Could you check a few things on this model? Use its own coordinates, in mm. A direction names the side the tool comes from. Coordinates: 2 decimals unless noted, no trailing zeros. Order: outer loops, then holes, each group sorted by start corner. A loop starts at its lowest first (then second) coordinate and runs counter-clockwise, first axis right, second up. Notation, with made-up numbers: (-29.75, -14.75) - (-5.75, -14.75) arc R16 cw to (-5.75, 9.25) - close; hole circle Ø1 at (87.25, 43). An arc over 180 degrees is marked (long way). One line per item, written item: value.
from build123d import *

# Parameters (mm, degrees)
SKETCH_1_R           = 1
EXTRUDE_1_DEPTH      = 4
EXTRUDE_START        = 4
SKETCH_2_R           = 1.732050808
EXTRUDE_2_DEPTH      = 5
EXTRUDE_3_DEPTH      = 0.75
EXTRUDE_3_DEPTH_BACK = 0.75
SKETCH_3_R           = 2.5


with BuildPart() as part:
    # 草图1 → 凸台-拉伸1 (new body)
    with BuildSketch(Plane.XY):
        Polygon((0.866025404, 1.5), (-0.866025404, 1.5), (-1.732050808, 0), (-0.866025404, -1.5), (0.866025404, -1.5), (1.732050808, 0), align=None)
        Circle(SKETCH_1_R, mode=Mode.SUBTRACT)
    extrude(amount=EXTRUDE_1_DEPTH)

    # 草图2 → 凸台-拉伸2 (add)
    with BuildSketch(Plane.XY.offset(EXTRUDE_START)):
        Circle(SKETCH_2_R)
    extrude(amount=EXTRUDE_2_DEPTH)

    # 草图3 → 凸台-拉伸3 (add, two sides: drawn at the far end of the back side and taken through both)
    with BuildSketch(Plane(origin=(0, 0, 0), x_dir=(1, 0, 0), z_dir=(0, 1, 0)).offset(-EXTRUDE_3_DEPTH_BACK)):
        with BuildLine():
            Line((-1.732050808, -9), (-3.661865884, -13.39042296))
            ThreePointArc((-3.661865884, -13.39042296), (0, -19), (3.661865884, -13.39042296))
            Line((3.661865884, -13.39042296), (1.732050808, -9))
            Line((1.732050808, -9), (-1.732050808, -9))
        make_face()
        with Locations(Location((0, -15, 0), (0, 0, 270))):
            Circle(SKETCH_3_R, mode=Mode.SUBTRACT)
    extrude(amount=EXTRUDE_3_DEPTH + EXTRUDE_3_DEPTH_BACK)

    # 草图4 → 切除-旋转2 (revolve, cut)
    with BuildSketch(Plane(origin=(0, 0, 0), x_dir=(0, 0, -1), z_dir=(1, 0, 0))):
        with BuildLine():
            Line((-15, -2.610076627), (-15, 2.610076627))
            ThreePointArc((-15, 2.610076627), (-17.610076627, 0), (-15, -2.610076627))
        make_face()
    revolve(axis=Axis((0, -2.610076627, 15), (0, 1, 0)), mode=Mode.SUBTRACT)


solid = part.part
Item 1: If I drill on probe 1 along Y at (x, z) = (0, 2); probe 2 along Z at (x, y) = (0.75, 0.25); probe 3 along X at (y, z) = (-0.6, 14), over which ranges is the centre line in solid material (lowest first)?
Conclusion:
probe 1: -1.5 to -1, 1 to 1.5
probe 2: 4 to 12.51, 17.49 to 18.93
probe 3: -3.87 to -2.34, 2.34 to 3.87
Item 2: I want a section at B-B on z = 15. Please give me the cut outline in (x, y).
Conclusion:
outline: (-4, -0.75) - (-2.5, -0.75) arc R2.61 cw to (-2.5, 0.75) - (-4, 0.75) - close; (2.5, -0.75) - (4, -0.75) - (4, 0.75) - (2.5, 0.75) arc R2.61 cw to start
Item 3: I want a section at A-A on x = 0. Please give me the cut outline in (y, z).
Conclusion:
outline: (-1.73, 4) - (-1.5, 4) - (-1.5, 0) - (-1, 0) - (-1, 4) - (1, 4) - (1, 0) - (1.5, 0) - (1.5, 4) - (1.73, 4) - (1.73, 9) - (0.75, 9) - (0.75, 12.5) arc R2.61 cw to (-0.75, 12.5) - (-0.75, 9) - (-1.73, 9) - close; (-0.75, 17.5) arc R2.61 cw to (0.75, 17.5) - (0.75, 19) - (-0.75, 19) - close
Item 4: I'm going to push flat-ended pins straight in: pin 1 Ø0.8 at (x, y) = (0.5, 1) entering from +Z; pin 2 Ø1.5 at (x, z) = (-2, 8.5) entering from -Y; pin 3 Ø3 at (x, z) = (1, 14.5) entering from -Y. Where does each tip first touch, or does it pass through?
Conclusion:
pin 1: z = 19
pin 2: y = -1.2
pin 3: y = -0.75
Item 5: Thinking about a two-plate mould opening in X: for faces 6 (the face through (0, -1, 2)), 7 (the face through (1.293, -0.76, 1.972)), 8 (the face through (0, 0, 4)), 9 (the face through (-0.38, -1.69, 6.46)), which applies, pulls with the +X half, pulls with the -X half, needs draft (parallel to the pull), parting line crosses it, or undercut?
Conclusion:
face 6: undercut
face 7: pulls with the +X half
face 8: undercut
face 9: parting line crosses it
Item 6: I want a section at D-D on y = -0.55. Please give me the cut outline in (x, z).
Conclusion:
outline: (-3.66, 13.39) - (-1.73, 9) - (-1.64, 9) - (-1.64, 4) - (-1.41, 4) - (-1.41, 0) - (-0.84, 0) - (-0.84, 4) - (0.84, 4) - (0.84, 0) - (1.41, 0) - (1.41, 4) - (1.64, 4) - (1.64, 9) - (1.73, 9) - (3.66, 13.39) arc R4 ccw (long way) to start; hole circle Ø5.1 at (0, 15)
Item 7: For faces 1 (the face through (2, -0.75, 13)), 2 (the face through (-1.305, -0.74, 1.972)), 3 (the face through (2, 0.75, 13)), 4 (the face through (1.305, 0.74, 1.972)), 5 (the face through (0, 1.5, 2)), which set-ups out of +Z, -Z, +X, -X, +Y, -Y let a thin tool reach every point of the face, with its end or its side?
Conclusion:
face 1: +Z, +X, -X, -Y
face 2: -Z, -X, -Y
face 3: +Z, +X, -X, +Y
face 4: -Z, +X, +Y
face 5: -Z, +X, -X, +Y
Item 8: I want a section at C-C on y = 1.25. Please give me the cut outline in (x, z).
Conclusion:
outline: (-1.2, 4) - (-1.01, 4) - (-1.01, 0) - (1.01, 0) - (1.01, 4) - (1.2, 4) - (1.2, 9) - (-1.2, 9) - close
